from build123d import *

# Parameters (mm, degrees)
BOSS_EXTRUDE1_DEPTH = 38.1


with BuildPart() as part:
    # Sketch1 → Boss-Extrude1 (new body)
    with BuildSketch(Plane.XY):
        with BuildLine():
            Line((33.170312314, -47.627428872), (93.967860133, -47.627428872))
            Line((93.967860133, -47.627428872), (93.967860133, -74.332818087))
            Line((93.967860133, -74.332818087), (-101.288011779, -74.332818087))
            Line((-101.288011779, -74.332818087), (-101.288011779, -47.627428872))
            Line((-101.288011779, -47.627428872), (-33.170312314, -47.627428872))
            ThreePointArc((-33.170312314, -47.627428872), (0, -58.04), (33.170312314, -47.627428872))
        make_face()
    extrude(amount=-BOSS_EXTRUDE1_DEPTH)


solid = part.part
For this review, take the finished solid that the model builds, in its own axes (mm). Coordinates: 2 decimals unless noted, no trailing zeros. Loops run counter-clockwise (first coordinate to the right, second up) from the corner with the lowest first, then second, coordinate; pieces in that order, holes last. Notation, with made-up numbers: (-8, 72.5) -> (27, 72.5) arc R19 cw to (27, 99.5) -> close; hole circle Ø8 at (-9, 28). An arc over 180 degrees is marked (long way). Write each question's results on one line, items separated by ' | '.
Q1. To check wall thickness, follow line 1 along Y through (x, z) = (-10.5, -2.5); line 2 along X through (y, z) = (-54, -12); line 3 along X through (y, z) = (-49.5, -16.5). State the ranges of each line that lie inside material, in increasing order. Write a range as [from, to].
Taken from the geometry:
line 1: [-74.33, -57.08] | line 2: [-101.29, -21.28], [21.28, 93.97] | line 3: [-101.29, -30.3], [30.3, 93.97]
Q2. Add section A-A, the plane y = -55.25. State the section outline as (x, z) points.
Taken from the geometry:
outline: (-101.29, -38.1) -> (-17.78, -38.1) -> (-17.78, 0) -> (-101.29, 0) -> close; (17.78, -38.1) -> (93.97, -38.1) -> (93.97, 0) -> (17.78, 0) -> close
Q3. Add section B-B, the plane z = -20. State the section outline as (x, y) points, then the cut area to 3 significant figures.
Taken from the geometry:
outline: (-101.29, -74.33) -> (93.97, -74.33) -> (93.97, -47.63) -> (33.17, -47.63) arc R58.04 cw to (-33.17, -47.63) -> (-101.29, -47.63) -> close | area: 4,740 mm²
Q4. Mouldability with a two-part tool opening along X and no side actions: class faces 1 (the flat face through (-101.288, -61, -19)), 2 (the cylindrical face through (-0.494, -58.038, -18.783)), 3 (the flat face through (-2, -61, 0)) as +X half, -X half, draft (parallel to the pull), parting line (faces both ways), or undercut.
Taken from the geometry:
face 1: -X half | face 2: undercut | face 3: draft
